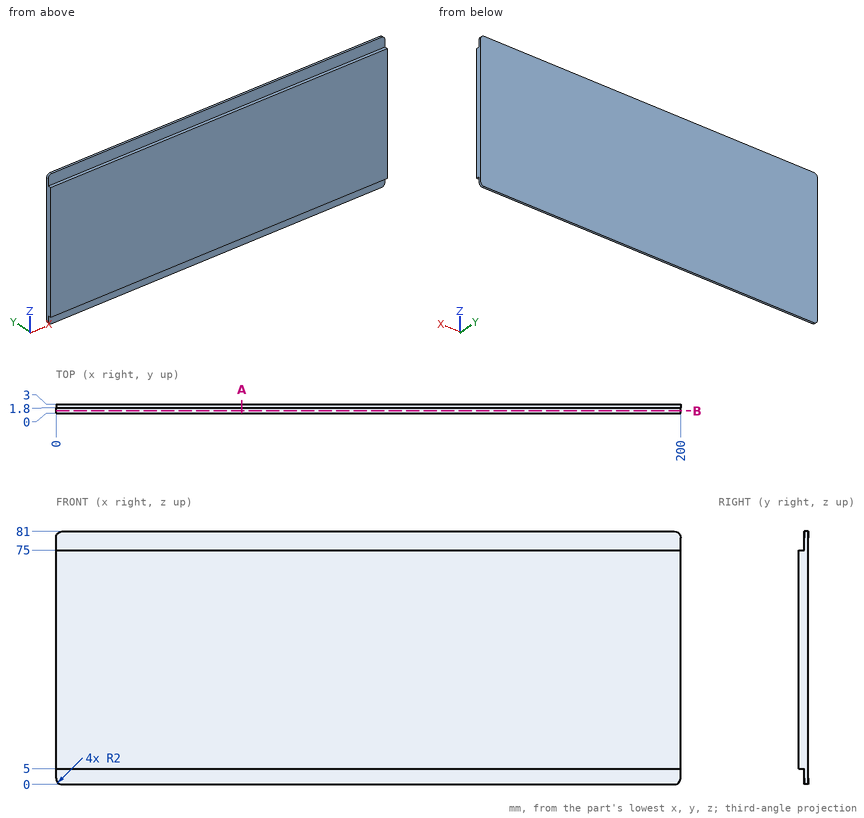
Check sheet for the drawn part. Datum: minimum x, y, z corner. Units: mm. Coordinates: 2 decimals unless noted, no trailing zeros. Order: outer loops, then holes, each group sorted by start corner. A loop starts at its lowest first (then second) coordinate and runs counter-clockwise, first axis right, second up. Notation, with made-up numbers: (13.5, 19.25) - (65.5, 19.25) arc R19 cw to (65.5, 45.25) - close; hole circle Ø7 at (-15.5, 61). An arc over 180 degrees is marked (long way). Return JSON: item names as keys, results as strings.
(1) Section check A-A, the plane x = 59.5. Record the cut outline in (y, z), and give its area (3 significant figures).
Filled sheet:
{"outline": "(0, 5) - (1.8, 5) - (1.8, 0) - (3, 0) - (3, 81) - (1.8, 81) - (1.8, 75) - (0, 75) - close", "area": "223 mm^2"}
(2) Thickness scan on line 1 along Z through (x, y) = (190, 0.95); line 2 along Y through (x, z) = (118, 4). Record the ranges inside material, lowest first.
Filled sheet:
{"line 1": "z = 5 to 75", "line 2": "y = 1.8 to 3"}
(3) Section check B-B, the plane y = 0.8. Record the cut outline in (x, z).
Filled sheet:
{"outline": "(0, 5) - (200, 5) - (200, 75) - (0, 75) - close"}
(4) Go/stop test with flat-tipped pins: pin 1 (1.5 mm diameter, centred on x = 86, z = 3, fed in from -Y); pin 2 (0.5 mm diameter, centred on x = 90.5, y = 0.5, fed in from +Z); pin 3 (1.4 mm diameter, centred on x = 113, y = 1, fed in from -Z). Record where each tip stops, or that it passes through.
Filled sheet:
{"pin 1": "stops at y = 1.8", "pin 2": "stops at z = 75", "pin 3": "stops at z = 5"}
